Input: part model. Units: mm. Frame: model coordinates. Round coordinates to 2 decimals unless told otherwise and drop trailing zeros. Order: outer loops, then holes, each group sorted by start corner. A loop starts at its lowest first (then second) coordinate and runs counter-clockwise, first axis right, second up.
Item 1: Cut plane B-B on z = 1166.5. Output: boundary loops of the cut face in (x, y).
Item 2: Cut plane A-A on y = 13. Output: boundary loops of the cut face in (x, z), then the cut area to 3 significant figures.
Item 3: Line query: L1, parallel to Z at x = 1, y = -23.9; L2, parallel to X at y = 22, z = 888; L3, parallel to Y at x = 8, z = 373. Output: solid intervals per line, ascending.
Item 4: First-contact query: pin 1 (9.5 mm diameter, centred on x = 1, z = 1228.5, fed in from -Y) (3 decimals). Flat tip, straight axial feed; report the tip coordinate or a pass-through.
Autodesk Inventor part; units mm, degrees
ref_plane "Start Plane" through (0, 0, 67.4996) normal (0, 0, 1) x (1, 0, 0)
ref_plane "End Plane" through (0, 0, 2247.5004) normal (0, 0, 1) x (1, 0, 0)
ref_plane "Work Plane4" through (-360.0026, 21, 2287.5) normal (0, 0, 1) x (1, 0, 0)
ref_plane "Start Plane" through (0, 0, 67.4996) normal (0, 0, 1) x (1, 0, 0)
ref_plane "End Plane" through (0, 0, 2247.5004) normal (0, 0, 1) x (1, 0, 0)
sketch "Sketch" plane through (0, 0, 0) normal (0, 0, 1) x (1, 0, 0)
  line L0 (-25, -21) -> (-25, 21)
  line L1 (-21, 25) -> (21, 25)
  line L2 (25, 21) -> (25, -21)
  line L3 (21, -25) -> (-21, -25)
  arc A0 (-25, -21) -> (-21, -25) centre (-21, -21) ccw
  arc A1 (25, 21) -> (21, 25) centre (21, 21) ccw
  arc A2 (-21, 25) -> (-25, 21) centre (-21, 21) ccw
  arc A3 (21, -25) -> (25, -21) centre (21, -21) ccw
  arc A4 (-21, 23) -> (-23, 21) centre (-21, 21) ccw
  line L4 (-21, 23) -> (21, 23)
  arc A5 (23, 21) -> (21, 23) centre (21, 21) ccw
  line L5 (23, 21) -> (23, -21)
  arc A6 (21, -23) -> (23, -21) centre (21, -21) ccw
  line L6 (21, -23) -> (-21, -23)
  arc A7 (-23, -21) -> (-21, -23) centre (-21, -21) ccw
  line L7 (-23, -21) -> (-23, 21)
  line L8 (0, 36.1598) -> (0, -36.1598) construction
  line L9 (-36.1598, 0) -> (36.1598, 0) construction
  dimension "d7" = 4
  dimension "d9" = 50
  dimension "d11" = 50
  dimension "d12" = 2
  dimension "d15" = 25
  dimension "d16" = 25
extrude "Body" add sketch "Sketch" along normal up to surface (2180.0008 mm away) from surface at 67.4996
sketch "Sketch3" plane through (0, 0, 0) normal (0, 0, 1) x (1, 0, 0)
  line L0 (0, 0) -> (10, 0)
ref_plane "Work Plane3" through (0, 0, 0) normal (0, -1, 0) x (1, 0, 0)
sketch "Sketch4" plane through (0, 0, 0) normal (0, -1, 0) x (1, 0, 0)
  line L0 (-2, 67.4996) -> (12, 67.4996)
  line L1 (-2, 2247.5004) -> (12, 2247.5004)
  dimension "d18" = 2180.0008
ref_plane "Work Plane4" through (-360.0026, 21, 2287.5) normal (0, 0, 1) x (1, 0, 0)
split "Split1" plane through (-360.0026, 21, 2287.5) removes the side toward (0, 0, 1)
ref_plane "Work Plane5" through (-360.0026, -21, 27.5) normal (0, 0, -1) x (-1, 0, 0)
split "Split2" plane through (-360.0026, -21, 27.5) removes the side toward (0, 0, -1)
sketch "Sketch5" plane through (21, 25, 2247.5004) normal (0, 1, 0) x (1, 0, 0)
  circle A0 centre (-20, 1019) radius 6
  circle A1 centre (-20, 1241.0001) radius 6
  point P0 (-21, 2247.5004)
extrude "Extrusion2" cut sketch "Sketch5" against normal through all
ref_plane "Work Plane6" through (-360.0026, -21, 67.5) normal (0, 0, -1) x (-1, 0, 0)
split "Split3" plane through (-360.0026, -21, 67.5) removes the side toward (0, 0, -1)
ref_plane "Work Plane7" through (-810.0026, 21, 2247.5) normal (0, 0, 1) x (1, 0, 0)
split "Split4" plane through (-810.0026, 21, 2247.5) removes the side toward (0, 0, 1)
equation "\"d7\" = G_IR"
equation "\"d9\" = G_W"
equation "\"d11\" = G_H"
equation "\"d12\" = G_T"
equation "\"d15\" = 0.5 * d9"
equation "\"d16\" = 0.5 * d11"
equation "\"d3\" = G_L"
equation "\"G_W\" = 50"
equation "\"G_H\" = 50"
equation "\"G_T\" = 2"
equation "\"G_IR\" = 4"
equation "\"G_L\" = d18"
equation "\"G_OFFSET_START\" = -67.49959"
equation "\"G_OFFSET_END\" = -67.49962"
equation "\"d13\" = -G_OFFSET_START"
equation "\"d14\" = G_OFFSET_END + B_L"
equation "\"B_L\" = 2315"
properties part number "ISO 10799-2 - 50x50x2 - 2180" material "Steel, Galvanized"
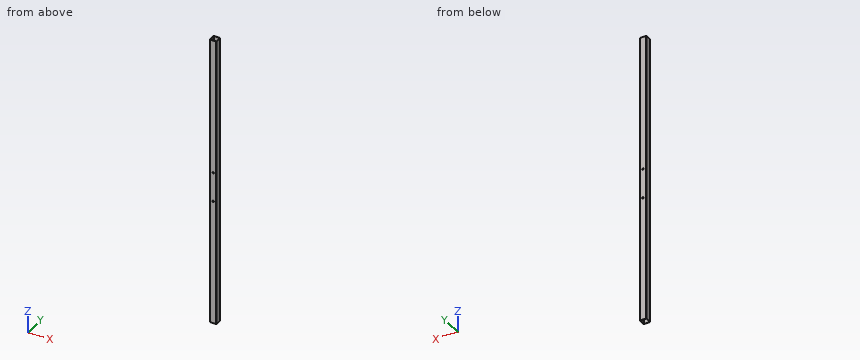
From the geometry:
1. outline: (-25, -21) arc R4 ccw to (-21, -25) - (21, -25) arc R4 ccw to (25, -21) - (25, 21) arc R4 ccw to (21, 25) - (-21, 25) arc R4 ccw to (-25, 21) - close; hole (-23, -21) arc R2 ccw to (-21, -23) - (21, -23) arc R2 ccw to (23, -21) - (23, 21) arc R2 ccw to (21, 23) - (-21, 23) arc R2 ccw to (-23, 21) - close
2. outline: (-25, 67.5) - (-23, 67.5) - (-23, 2247.5) - (-25, 2247.5) - close; (23, 67.5) - (25, 67.5) - (25, 2247.5) - (23, 2247.5) - close
2. area: 8,720 mm2
3. L1: z = 67.5 to 1000.5, 1012.5 to 1222.5, 1234.5 to 2247.5
3. L2: x = -24.87 to -22.73, 22.73 to 24.87
3. L3: y = -25 to -23, 23 to 25
4. pin 1: passes through
